```python
from build123d import *


with BuildPart() as part:
    # 草图1 → 旋转1 (revolve)
    with BuildSketch(Plane(origin=(0, 0, 0), x_dir=(1, 0, 0), z_dir=(0, 1, 0)), mode=Mode.PRIVATE) as revolve_1_sk:
        Polygon((20.5, 0), (20.5, 10), (28, 10), (28, 5), (25.5, 5), (25.5, 4), (26, 4), (26, 0), align=None)
    revolve(revolve_1_sk.sketch.rotate(Axis((0, 0, -19.14057971), (0, 0, 1)), 180), axis=Axis((0, 0, -19.14057971), (0, 0, 1)))  # turned: the seam where the file's is


solid = part.part
```
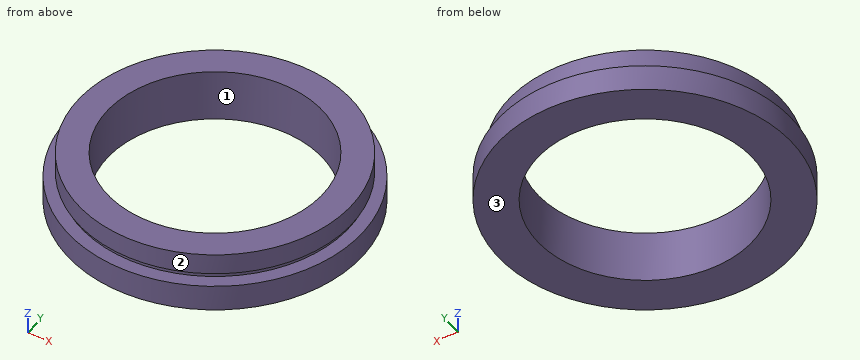
Geometry: final body of the model. Coordinates: model frame, mm. Face numbers are marked on the shaded views. Round coordinates to 2 decimals unless told otherwise and drop trailing zeros. Order: outer loops, then holes, each group sorted by start corner. A loop starts at its lowest first (then second) coordinate and runs counter-clockwise, first axis right, second up. Notation, with made-up numbers: (10.25, 57) -> (43.25, 57) arc R15 cw to (43.25, 71) -> close; hole circle Ø9 at (-40, 34.5). An arc over 180 degrees is marked (long way). Use CSV: the item, a comma, the result in double quotes. Start each with the question number.
1) Material intervals for line 1 along Z through (x, y) = (-21, -15); line 2 along Y through (x, z) = (-17, -2.75); line 3 along Y through (x, z) = (0, -2.25), sorted ascending. Write a range as from..to.
2) Section A-A (x = 0). Return the cut outline in (y, z).
3) First-contact query: pin 1 Ø5 at (x, z) = (21.5, -1) entering from -Y; pin 2 Ø5 at (y, z) = (-18.5, -3.5) entering from -X; pin 3 Ø4 at (x, z) = (-2, -5.5) entering from +Y. Flat tips, straight axial feed; report the tip coordinate or a pass-through.
4) Section C-C (z = -7.75). Return the cut outline in (x, y).
5) Section D-D (x = 24). Return the cut outline in (y, z), and give its area (3 significant figures).
6) Draft query along Y for the marked faces 1, 2 and 3. Return one class per face: +Y half, -Y half, draft (parallel to the pull), parting line (faces both ways), or undercut.
Returned:
1,line 1,"z = -10..-5, -4..0"
1,line 2,"y = -19.67..-11.46, 11.46..19.67"
1,line 3,"y = -26..-20.5, 20.5..26"
2,outline,"(-28, -10) -> (-20.5, -10) -> (-20.5, 0) -> (-26, 0) -> (-26, -4) -> (-25.5, -4) -> (-25.5, -5) -> (-28, -5) -> close; (20.5, -10) -> (28, -10) -> (28, -5) -> (25.5, -5) -> (25.5, -4) -> (26, -4) -> (26, 0) -> (20.5, 0) -> close"
3,pin 1,"stops at y = -17.75"
3,pin 2,"stops at x = -22.62"
3,pin 3,"stops at y = 28"
4,outline,"circle Ø56 at (0, 0); hole circle Ø41 at (0, 0)"
5,outline,"(-14.42, -10) -> (14.42, -10) -> (14.42, -5) -> (8.62, -5) -> (8.62, -4) -> (10, -4) -> (10, 0) -> (-10, 0) -> (-10, -4) -> (-8.62, -4) -> (-8.62, -5) -> (-14.42, -5) -> close"
5,area,"241 mm²"
6,face 1,"undercut"
6,face 2,"parting line"
6,face 3,"draft"
